Geometry: final body of the model. Coordinates: model frame, mm. Face numbers are marked on the shaded views. A direction names the side the tool comes from. Coordinates: 2 decimals unless noted, no trailing zeros. Write each loop counter-clockwise with the first axis right and the second up, starting at its lowest first coordinate (ties: lowest second). Pieces come first, ordered by that corner, then holes.
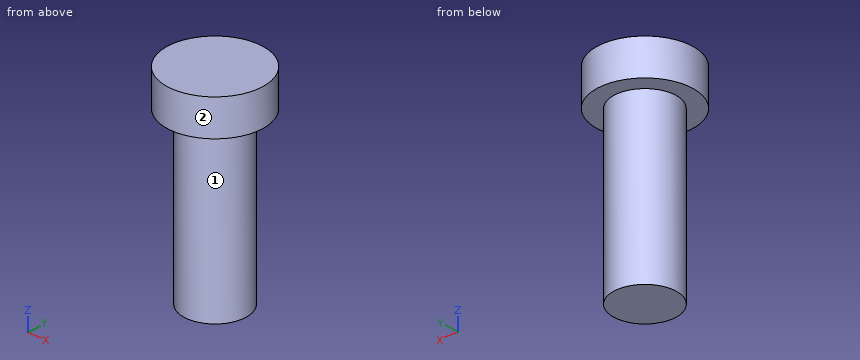
from build123d import *

# Parameters (mm, degrees)
CYLINDER004_R     = 2.6
CYLINDER004_DEPTH = 14
CYLINDER003_R     = 4
CYLINDER003_DEPTH = 3


with BuildPart() as button_pusher:
    # Cylinder004 → Cylinder004 (new body)
    with BuildSketch(Plane.XY):
        Circle(CYLINDER004_R)
    extrude(amount=CYLINDER004_DEPTH)


with BuildPart() as button_pusher_fusion:
    # Cylinder003 → Cylinder003 (new body)
    with BuildSketch(Plane.XY.offset(14)):
        Circle(CYLINDER003_R)
    extrude(amount=CYLINDER003_DEPTH)

    # Fusion009: union button pusher
    add(button_pusher.part)


solid = button_pusher_fusion.part
Item 1: Section C-C, the plane z = 3.75. Output: boundary loops of the cut face in (x, y).
Derived:
outline: circle Ø5.2 at (0, 0)
Item 2: Section A-A, the plane y = 0. Output: boundary loops of the cut face in (x, z), plus the area to 3 significant figures.
Derived:
outline: (-4, 14) - (-2.6, 14) - (-2.6, 0) - (2.6, 0) - (2.6, 14) - (4, 14) - (4, 17) - (-4, 17) - close
area: 96.8 mm2
Item 3: Material intervals for probe 1 along Z at (x, y) = (-3, 0.75); probe 2 along X at (y, z) = (2.25, 11.25); probe 3 along X at (y, z) = (1.5, 5.5), sorted ascending.
Derived:
probe 1: z = 14 to 17
probe 2: x = -1.3 to 1.3
probe 3: x = -2.12 to 2.12
Item 4: Pin query (flat end, axial travel): pin 1 (3 mm diameter, centred on y = 0.5, z = 6, fed in from -X). Return the tip coordinate at first contact, or that it passes through.
Derived:
pin 1: stops at x = -2.6
Item 5: Set-up query: the marked faces 1 and 2. Return all of +Z, -Z, +X, -X, +Y, -Y with unobstructed straight access to the full face (end or side cutting, diameter ignored); none if empty.
Derived:
face 1: -Z
face 2: +Z, -Z
Item 6: Section D-D, the plane x = -3.5. Output: boundary loops of the cut face in (y, z), plus the area to 3 significant figures.
Derived:
outline: (-1.94, 14) - (1.94, 14) - (1.94, 17) - (-1.94, 17) - close
area: 11.6 mm2
